```python
from build123d import *

# Parameters (mm, degrees)
BOSS_EXTRUDE1_DEPTH = 146.05
FILLET2_R           = 0.254
FILLET1_R           = 1.27
SKETCH5_W           = 7.112
SKETCH5_H           = 2.54
BOSS_EXTRUDE2_DEPTH = 292.1


with BuildPart() as part:
    # Sketch3 → Boss-Extrude1 (new body, symmetric)
    with BuildSketch(Plane.XY):
        with BuildLine():
            Line((-12.7, 12.7), (-1.796051224, 1.796051224))
            ThreePointArc((-1.796051224, 1.796051224), (-0.972015918, 2.346654013), (0, 2.54))
            Line((0, 2.54), (0, 4.826))
            Line((0, 4.826), (-1.977846327, 4.826))
            ThreePointArc((-1.977846327, 4.826), (-2.949862246, 5.019345987), (-3.773897552, 5.569948776))
            Line((-3.773897552, 5.569948776), (-7.772528286, 9.56857951))
            ThreePointArc((-7.772528286, 9.56857951), (-7.847628361, 9.946133082), (-7.527553898, 10.16))
            Line((-7.527553898, 10.16), (-3.302, 10.16))
            Line((-3.302, 10.16), (-3.302, 12.7))
            Line((-3.302, 12.7), (-12.7, 12.7))
        make_face()
    extrude(amount=BOSS_EXTRUDE1_DEPTH, both=True)

    # Fillet2
    fillet2_edges = [part.edges().sort_by_distance(p)[0] for p in [
        (-3.302, 12.7, 0),
        (-3.302, 10.16, 0),
    ]]
    fillet(fillet2_edges, radius=FILLET2_R)

    # Mirror1: part across plane


with BuildPart() as part_1:
    add(part.part)
    add(part.part.mirror(Plane(origin=(0, 0, 146.05), x_dir=(0, 0, 1), z_dir=(0.707106781, 0.707106781, 0))))

    # Fillet1
    fillet1_edges = [part_1.edges().sort_by_distance(p)[0] for p in [
        (-12.7, 12.7, 0),
    ]]
    fillet(fillet1_edges, radius=FILLET1_R)

    # Mirror2: part across plane


with BuildPart() as part_2:
    add(part_1.part)
    add(part_1.part.mirror(Plane(origin=(0, 0, 146.05), x_dir=(0, 0, 1), z_dir=(0, 1, 0))))

    # Mirror5: part across plane


with BuildPart() as part_3:
    add(part_2.part)
    add(part_2.part.mirror(Plane(origin=(0, 0, 146.05), x_dir=(0, 0, 1), z_dir=(-1, 0, 0))))

    # Sketch5 → Boss-Extrude2 (add, through all)
    with BuildSketch(Plane.XY.offset(146.05)):
        with Locations((0, -11.43)):
            Rectangle(SKETCH5_W, SKETCH5_H)
    extrude(amount=-BOSS_EXTRUDE2_DEPTH)


solid = part_3.part
```
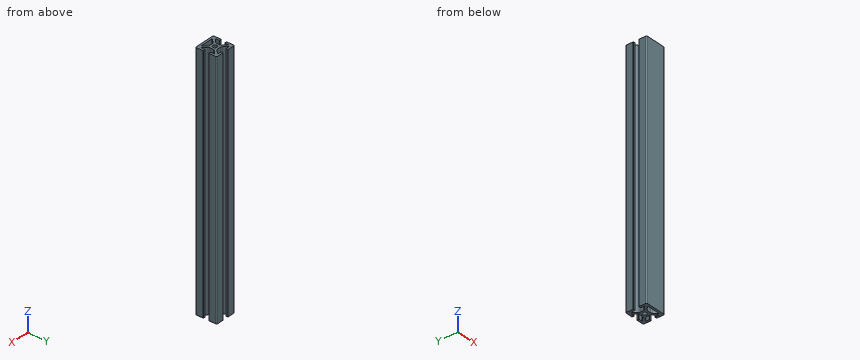
Could you check a few things on this model? Use its own coordinates, in mm. Round coordinates to 2 decimals unless told otherwise and drop trailing zeros.
(1) If I drill on probe 1 along X at (y, z) = (3.75, 69.5); probe 2 along X at (y, z) = (0.5, 119.5), over which ranges is the centre line in solid material (lowest first)?
Findings below:
probe 1: x = -12.7 to -10.16, -5.55 to 5.55, 10.16 to 12.7
probe 2: x = -4.83 to -2.49, 2.49 to 4.83
(2) For pin 1 (3 mm diameter, centred on y = 0, z = 42, fed in from -X); pin 2 (1.2 mm diameter, centred on x = 0.5, z = -62, fed in from +Y); pin 3 (1.2 mm diameter, centred on y = 1, z = -20, fed in from +X), each with a flat end and sliding along its axis, tell me the tip position at first contact or that it passes through.
Findings below:
pin 1: stops at x = -4.83
pin 2: stops at y = 4.83
pin 3: stops at x = 4.83
(3) Suppose I cut it at A-A on z = -58.5. State how many separate pieces and enclosed holes the cut face has, and give its area (3 significant figures).
Findings below:
separate pieces: 1
enclosed holes: 2
area: 332 mm2
